Drawing for the job (mm, zero at the part's lowest x, y, z). A direction names the side the tool comes from. Coordinates: 2 decimals unless noted, no trailing zeros. Write each loop counter-clockwise with the first axis right and the second up, starting at its lowest first coordinate (ties: lowest second). Pieces come first, ordered by that corner, then holes. Notation, with made-up numbers: (-21, 68.5) -> (-8, 68.5) arc R22 cw to (-8, 79.5) -> close; hole circle Ø4 at (-11.5, -37). An arc over 180 degrees is marked (long way). Write item = value, one per line. Start each with the question number.
Q1. Tool access for the marked faces 1 and 2: list every direction of +Z, -Z, +X, -X, +Y, -Y with a clear straight run to the whole face (end or side of a thin tool).
Q2. Pull direction X, two halves, no side cores. Call the marked faces 3, 4 and 5: released by +X, released by -X, zero draft, split by the parting line, or undercut.
Q3. Band-saw the part on A-A, the plane y = 1.75. List the corners of the cut face in (x, z), plus the area to 3 significant figures.
Q4. Band-saw the part on C-C, the plane x = 30. List the corners of the cut face in (y, z), plus the area to 3 significant figures.
Q5. Band-saw the part on B-B, the plane z = 36. List the corners of the cut face in (x, y), plus the area to 3 significant figures.
Q6. Pin check, flat tip, straight feed: P1, Ø9.5, axis at x = 65, z = 26, coming from the -Y side. Stop position of the tip, or through.
Q7. Probe line 1 (X direction, y = 3.75, z = 35); line 2 (Z direction, x = 104, y = 1.25); line 3 (Y direction, x = 77.5, z = 11). List the from-to ranges inside material, lowest first.
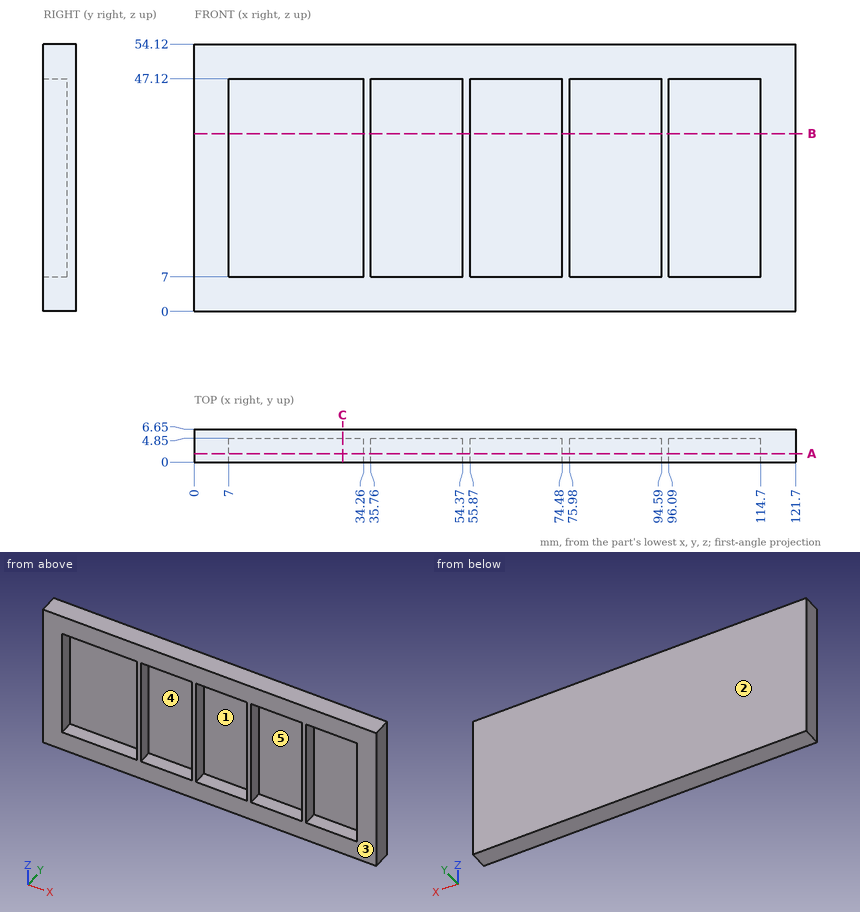
Ans:
q1.face_1 = -Y
q1.face_2 = +Z, -Z, +X, -X, +Y
q2.face_3 = zero draft
q2.face_4 = undercut
q2.face_5 = undercut
q3.outline = (0, 0) -> (121.7, 0) -> (121.7, 54.12) -> (0, 54.12) -> close; hole (7, 7) -> (34.26, 7) -> (34.26, 47.12) -> (7, 47.12) -> close; hole (35.76, 7) -> (54.37, 7) -> (54.37, 47.12) -> (35.76, 47.12) -> close; hole (55.87, 7) -> (74.48, 7) -> (74.48, 47.12) -> (55.87, 47.12) -> close; hole (75.98, 7) -> (94.59, 7) -> (94.59, 47.12) -> (75.98, 47.12) -> close; hole (96.09, 7) -> (114.7, 7) -> (114.7, 47.12) -> (96.09, 47.12) -> close
q3.area = 2,510 mm2
q4.outline = (0, 0) -> (6.65, 0) -> (6.65, 54.12) -> (0, 54.12) -> (0, 47.12) -> (4.85, 47.12) -> (4.85, 7) -> (0, 7) -> close
q4.area = 165 mm2
q5.outline = (0, 0) -> (7, 0) -> (7, 4.85) -> (34.26, 4.85) -> (34.26, 0) -> (35.76, 0) -> (35.76, 4.85) -> (54.37, 4.85) -> (54.37, 0) -> (55.87, 0) -> (55.87, 4.85) -> (74.48, 4.85) -> (74.48, 0) -> (75.98, 0) -> (75.98, 4.85) -> (94.59, 4.85) -> (94.59, 0) -> (96.09, 0) -> (96.09, 4.85) -> (114.7, 4.85) -> (114.7, 0) -> (121.7, 0) -> (121.7, 6.65) -> (0, 6.65) -> close
q5.area = 316 mm2
q6.P1 = 4.85
q7.line_1 = 0 to 7, 34.26 to 35.76, 54.37 to 55.87, 74.48 to 75.98, 94.59 to 96.09, 114.7 to 121.7
q7.line_2 = 0 to 7, 47.12 to 54.12
q7.line_3 = 4.85 to 6.65
